```python
from build123d import *

# Parameters (mm, degrees)
SKETCH2_W           = 85
SKETCH2_H           = 66.5
BOSS_EXTRUDE2_DEPTH = 3
SKETCH3_W           = 85
SKETCH3_H           = 66.5
SKETCH3_W_2         = 79
SKETCH3_H_2         = 60.5
SKETCH3_H_3         = 8
BOSS_EXTRUDE3_DEPTH = 4
SKETCH4_R           = 2
CUT_EXTRUDE1_DEPTH  = 4.5
SKETCH5_W           = 85
SKETCH5_H           = 66.5
SKETCH5_W_2         = 79
SKETCH5_H_2         = 60.5
BOSS_EXTRUDE4_DEPTH = 1.6
BOSS_EXTRUDE5_START = -8.6
SKETCH6_W           = 10
SKETCH6_H           = 10
BOSS_EXTRUDE5_DEPTH = 8.6
CUT_EXTRUDE2_DEPTH  = 4.5
FILLET1_R           = 2


with BuildPart() as part:
    # Sketch2 → Boss-Extrude2 (new body)
    with BuildSketch(Plane(origin=(0, 0, 0), x_dir=(1, 0, 0), z_dir=(0, 1, 0))):
        Rectangle(SKETCH2_W, SKETCH2_H)
    extrude(amount=BOSS_EXTRUDE2_DEPTH)

    # Sketch3 → Boss-Extrude3 (add)
    # profile 1 of 3: a face of its own
    with BuildSketch(Plane(origin=(0, 3, 0), x_dir=(1, 0, 0), z_dir=(0, 1, 0))):
        Rectangle(SKETCH3_W, SKETCH3_H)
        Rectangle(SKETCH3_W_2, SKETCH3_H_2, mode=Mode.SUBTRACT)
    # profile 2 of 3: a face of its own
    with BuildSketch(Plane(origin=(0, 3, 0), x_dir=(1, 0, 0), z_dir=(0, 1, 0))):
        with Locations((0, 26.25)):
            Rectangle(SKETCH3_W_2, SKETCH3_H_3)
    # profile 3 of 3: a face of its own
    with BuildSketch(Plane(origin=(0, 3, 0), x_dir=(1, 0, 0), z_dir=(0, 1, 0))):
        with Locations((0, -26.25)):
            Rectangle(SKETCH3_W_2, SKETCH3_H_3)
    extrude(amount=BOSS_EXTRUDE3_DEPTH)

    # Sketch4 → Cut-Extrude1 (cut)
    with BuildSketch(Plane(origin=(0, 7, 0), x_dir=(1, 0, 0), z_dir=(0, 1, 0))):
        with Locations(Location((-35.89, 26.3, 0), (0, 0, 270))):
            Circle(SKETCH4_R)
        with Locations(Location((-35.89, -26.3, 0), (0, 0, 270))):
            Circle(SKETCH4_R)
        with Locations(Location((35.89, 26.3, 0), (0, 0, 270))):
            Circle(SKETCH4_R)
        with Locations(Location((32.89, -26.69684774, 0), (0, 0, 270))):
            Circle(SKETCH4_R)
    extrude(amount=-CUT_EXTRUDE1_DEPTH, mode=Mode.SUBTRACT)

    # Sketch5 → Boss-Extrude4 (add)
    with BuildSketch(Plane(origin=(0, 7, 0), x_dir=(1, 0, 0), z_dir=(0, 1, 0))):
        Rectangle(SKETCH5_W, SKETCH5_H)
        Rectangle(SKETCH5_W_2, SKETCH5_H_2, mode=Mode.SUBTRACT)
    extrude(amount=BOSS_EXTRUDE4_DEPTH)

    # Sketch6 → Boss-Extrude5 (add)
    with BuildSketch(Plane.XZ.offset(BOSS_EXTRUDE5_START)):
        with Locations((-37.5, -38.25)):
            Rectangle(SKETCH6_W, SKETCH6_H)
        with Locations((37.5, -38.25)):
            Rectangle(SKETCH6_W, SKETCH6_H)
        with Locations((37.5, 38.25)):
            Rectangle(SKETCH6_W, SKETCH6_H)
        with Locations((-37.5, 38.25)):
            Rectangle(SKETCH6_W, SKETCH6_H)
    extrude(amount=BOSS_EXTRUDE5_DEPTH)

    # Sketch7 → Cut-Extrude2 (cut)
    with BuildSketch(Plane(origin=(0, 8.6, 0), x_dir=(1, 0, 0), z_dir=(0, 1, 0))):
        with BuildLine():
            ThreePointArc((-38.914213562, 39.664213562), (-38.914213562, 36.835786438), (-36.085786438, 36.835786438))
            Line((-36.085786438, 36.835786438), (-38.914213562, 39.664213562))
        make_face()
        with BuildLine():
            Line((-38.914213562, 39.664213562), (-36.085786438, 36.835786438))
            ThreePointArc((-36.085786438, 36.835786438), (-35.652240935, 37.484633135), (-35.5, 38.25))
            ThreePointArc((-35.5, 38.25), (-36.734633135, 40.097759065), (-38.914213562, 39.664213562))
        make_face()
        with BuildLine():
            ThreePointArc((38.914213562, 39.664213562), (36.085786438, 39.664213562), (36.085786438, 36.835786438))
            Line((36.085786438, 36.835786438), (38.914213562, 39.664213562))
        make_face()
        with BuildLine():
            Line((38.914213562, 39.664213562), (36.085786438, 36.835786438))
            ThreePointArc((36.085786438, 36.835786438), (38.265366865, 36.402240935), (39.5, 38.25))
            ThreePointArc((39.5, 38.25), (39.347759065, 39.015366865), (38.914213562, 39.664213562))
        make_face()
        with BuildLine():
            ThreePointArc((39.5, -38.25), (38.265366865, -36.402240935), (36.085786438, -36.835786438))
            Line((36.085786438, -36.835786438), (38.914213562, -39.664213562))
            ThreePointArc((38.914213562, -39.664213562), (39.347759065, -39.015366865), (39.5, -38.25))
        make_face()
        with BuildLine():
            Line((38.914213562, -39.664213562), (36.085786438, -36.835786438))
            ThreePointArc((36.085786438, -36.835786438), (36.085786438, -39.664213562), (38.914213562, -39.664213562))
        make_face()
        with BuildLine():
            ThreePointArc((-36.085786438, -36.835786438), (-38.914213562, -36.835786438), (-38.914213562, -39.664213562))
            Line((-38.914213562, -39.664213562), (-36.085786438, -36.835786438))
        make_face()
        with BuildLine():
            Line((-36.085786438, -36.835786438), (-38.914213562, -39.664213562))
            ThreePointArc((-38.914213562, -39.664213562), (-36.734633135, -40.097759065), (-35.5, -38.25))
            ThreePointArc((-35.5, -38.25), (-35.652240935, -37.484633135), (-36.085786438, -36.835786438))
        make_face()
    extrude(amount=-CUT_EXTRUDE2_DEPTH, mode=Mode.SUBTRACT)

    # Fillet1
    fillet1_edges = [part.edges().sort_by_distance(p)[0] for p in [
        (42.5, 4.3, -43.25),
        (32.5, 4.3, -43.25),
        (32.5, 4.3, -33.25),
        (42.5, 4.3, 43.25),
        (32.5, 4.3, 33.25),
        (32.5, 4.3, 43.25),
        (-42.5, 4.3, 43.25),
        (-32.5, 4.3, 43.25),
        (-32.5, 4.3, 33.25),
        (-42.5, 4.3, -43.25),
        (-32.5, 4.3, -33.25),
        (-32.5, 4.3, -43.25),
    ]]
    fillet(fillet1_edges, radius=FILLET1_R)


solid = part.part
```
Input: part model. Units: mm. Frame: model coordinates. A direction names the side the tool comes from. Give positions to 0.01 mm unless a question says otherwise; leave off trailing zeros. Write each loop counter-clockwise with the first axis right and the second up, starting at its lowest first coordinate (ties: lowest second). Pieces come first, ordered by that corner, then holes. Notation, with made-up numbers: (-30, -37.5) - (4, -37.5) arc R7 ccw to (4, -30.5) - close; hole circle Ø10 at (-20.5, 19). An arc over 180 degrees is marked (long way). Write item = value, one per line. Start each with the question number.
1. Mould query, pull axis X, two halves, no side actions, for faces 1 (the flat face through (0, 8.6, 32)), 2 (the cylindrical face through (-41.93, 4.24, 42.65)), 3 (the flat face through (-1, 3, 0)), 4 (the cylindrical face through (37.576, 4.781, -25.225)). Classes: released by +X, released by -X, zero draft, split by the parting line, or undercut.
2. Section query B-B, the plane x = -5.5. Output: boundary loops of the cut face in (y, z), then the cut area to 3 significant figures.
3. Access query for faces 5 (the flat face through (0, 4, 33.25)), 6 (the flat face through (-1, 0, 1)), 7 (the flat face through (-39.5, 6, 0)), 8 (the cylindrical face through (31.9, 4.24, -33.82)). Directions: +Z, -Z, +X, -X, +Y, -Y. A direction counts if a zero-diameter tool reaches every point of the face in a straight line with its end or side. Return the directions, or none.
4. First-contact query: pin 1 Ø1.8 at (x, y) = (-7.5, 8) entering from +Z; pin 2 Ø1.8 at (x, y) = (-7.5, 8) entering from -Z; pin 3 Ø3 at (x, z) = (-36, 27) entering from +Y. Flat tips, straight axial feed; report the tip coordinate or a pass-through.
5. Section query A-A, the plane z = -26.3. Output: boundary loops of the cut face in (x, y).
6. Ray query, L1, parallel to X at y = 6.5, z = 38; L2, parallel to X at y = 5.3, z = -26.3; L3, parallel to Z at x = -13, y = 4. Return the intervals inside material, ascending.
7. Section query D-D, the plane z = 20.5. Output: boundary loops of the cut face in (x, y), then the cut area to 3 significant figures.
8. Section query C-C, the plane y = 5.25. Count the separate pieces of the cut face and the enclosed holes in it, then the cut area to 3 significant figures.
Check sheet entries:
q1.face_1 = zero draft
q1.face_2 = released by -X
q1.face_3 = undercut
q1.face_4 = undercut
q2.outline = (0, -33.25) - (8.6, -33.25) - (8.6, -30.25) - (7, -30.25) - (7, -22.25) - (3, -22.25) - (3, 22.25) - (7, 22.25) - (7, 30.25) - (8.6, 30.25) - (8.6, 33.25) - (0, 33.25) - close
q2.area = 297 mm2
q3.face_5 = +Z, +Y, -Y
q3.face_6 = +Z, -Z, +X, -X, -Y
q3.face_7 = +Y
q3.face_8 = -Z, +Y, -Y
q4.pin_1 = 33.25
q4.pin_2 = -33.25
q4.pin_3 = 7
q5.outline = (-42.5, 0) - (42.5, 0) - (42.5, 8.6) - (39.5, 8.6) - (39.5, 7) - (37.89, 7) - (37.89, 2.5) - (33.89, 2.5) - (33.89, 7) - (-33.89, 7) - (-33.89, 2.5) - (-37.89, 2.5) - (-37.89, 7) - (-39.5, 7) - (-39.5, 8.6) - (-42.5, 8.6) - close
q6.L1 = -42.5 to -39.48, -35.52 to -32.5, 32.5 to 35.52, 39.48 to 42.5
q6.L2 = -42.5 to -37.89, -33.89 to 33.89, 37.89 to 42.5
q6.L3 = -33.25 to -22.25, 22.25 to 33.25
q7.outline = (-42.5, 0) - (42.5, 0) - (42.5, 8.6) - (39.5, 8.6) - (39.5, 3) - (-39.5, 3) - (-39.5, 8.6) - (-42.5, 8.6) - close
q7.area = 289 mm2
q8.separate_pieces = 1
q8.enclosed_holes = 9
q8.area = 2,430 mm2
